from build123d import *

# Parameters (mm, degrees)
SKETCH_1_W          = 48
SKETCH_1_H          = 22
EXTRUDE_1_DEPTH     = 6
SKETCH_4_W          = 46
SKETCH_4_H          = 4
CUT_EXTRUDE_2_DEPTH = 22
SKETCH_5_W          = 42
SKETCH_5_H          = 1
CUT_EXTRUDE_3_DEPTH = 22
SKETCH_9_W          = 12
SKETCH_9_H          = 4.5
CUT_EXTRUDE_5_DEPTH = 6
SKETCH_10_W         = 6
SKETCH_10_H         = 3
EXTRUDE_2_DEPTH     = 6
SKETCH_11_W         = 6
SKETCH_11_H         = 3
EXTRUDE_3_DEPTH     = 6
SKETCH_12_R         = 1.5
CUT_EXTRUDE_6_DEPTH = 3
SKETCH_14_R         = 1.5
CUT_EXTRUDE_7_DEPTH = 3


with BuildPart() as part:
    # 草圖1 → 填料-伸長1 (new body)
    with BuildSketch(Plane.XY):
        with Locations((-24, -11)):
            Rectangle(SKETCH_1_W, SKETCH_1_H)
    extrude(amount=EXTRUDE_1_DEPTH)

    # 草圖4 → 除料-伸長2 (cut)
    with BuildSketch(Plane(origin=(0, 0, 0), x_dir=(1, 0, 0), z_dir=(0, 1, 0))):
        with Locations((-24, -3)):
            Rectangle(SKETCH_4_W, SKETCH_4_H)
    extrude(amount=-CUT_EXTRUDE_2_DEPTH, mode=Mode.SUBTRACT)

    # 草圖5 → 除料-伸長3 (cut)
    with BuildSketch(Plane(origin=(0, 0, 0), x_dir=(1, 0, 0), z_dir=(0, 1, 0))):
        with Locations((-24, -0.5)):
            Rectangle(SKETCH_5_W, SKETCH_5_H)
    extrude(amount=-CUT_EXTRUDE_3_DEPTH, mode=Mode.SUBTRACT)

    # 草圖9 → 除料-伸長5 (cut)
    with BuildSketch(Plane.XY.offset(6)):
        with Locations((-24, -19.75)):
            Rectangle(SKETCH_9_W, SKETCH_9_H)
    extrude(amount=-CUT_EXTRUDE_5_DEPTH, mode=Mode.SUBTRACT)

    # 草圖10 → 填料-伸長2 (add)
    with BuildSketch(Plane(origin=(0, 0, 0), x_dir=(0, 0, -1), z_dir=(1, 0, 0))):
        with Locations((-3, -20.5)):
            Rectangle(SKETCH_10_W, SKETCH_10_H)
    extrude(amount=EXTRUDE_2_DEPTH)

    # 草圖11 → 填料-伸長3 (add)
    with BuildSketch(Plane.ZY.offset(48)):
        with Locations((3, -20.5)):
            Rectangle(SKETCH_11_W, SKETCH_11_H)
    extrude(amount=EXTRUDE_3_DEPTH)

    # 草圖12 → 除料-伸長6 (cut)
    with BuildSketch(Plane(origin=(0, -19, 0), x_dir=(1, 0, 0), z_dir=(0, 1, 0))):
        with Locations(Location((3, -3, 0), (0, 0, 180))):
            Circle(SKETCH_12_R)
    extrude(amount=-CUT_EXTRUDE_6_DEPTH, mode=Mode.SUBTRACT)

    # 草圖14 → 除料-伸長7 (cut)
    with BuildSketch(Plane(origin=(0, -19, 0), x_dir=(1, 0, 0), z_dir=(0, 1, 0))):
        with Locations(Location((-51, -3, 0), (0, 0, 270))):
            Circle(SKETCH_14_R)
    extrude(amount=-CUT_EXTRUDE_7_DEPTH, mode=Mode.SUBTRACT)


solid = part.part
Work out the finished part from the listing and answer in its coordinate system (mm). A direction names the side the tool comes from. Give positions to 0.01 mm unless a question says otherwise; leave off trailing zeros. Order: outer loops, then holes, each group sorted by start corner. A loop starts at its lowest first (then second) coordinate and runs counter-clockwise, first axis right, second up. Notation, with made-up numbers: M -34,-11 L -21,-11 A34 cw -21,22 Z; hole C -1,2.5 d1. An arc over 180 degrees is marked long. Return JSON: item names as keys, results as strings.
Q1. The mould has two halves that part along Z. Classify faces 4 (the face through (-47, -14, 0)), 5 (the face through (-2, -11, 1)), 6 (the face through (-47, -11, 3)), 7 (the face through (-27.7, 0, 5.4)): pulls with the +Z half, pulls with the -Z half, needs draft (parallel to the pull), parting line crosses it, or undercut.
Answer below:
{"face 4": "pulls with the -Z half", "face 5": "undercut", "face 6": "undercut", "face 7": "needs draft"}
Q2. Find the intervals of material crossed by line 1 along X through (y, z) = (-19.75, 3.1); line 2 along X through (y, z) = (-15.25, 1.4); line 3 along Z through (x, y) = (-1.5, -3.25), in increasing order. Write a range as [from, to].
Answer below:
{"line 1": "x = [-54, -52.5], [-49.5, -47], [-1, 1.5], [4.5, 6]", "line 2": "x = [-48, -47], [-1, 0]", "line 3": "z = [0, 1], [5, 6]"}
Q3. Find section C-C, the plane y = -5. Write down the section's boundary in (x, z), and give its area (3 significant figures).
Answer below:
{"outline": "M -48,0 L -45,0 L -45,1 L -47,1 L -47,5 L -1,5 L -1,1 L -3,1 L -3,0 L 0,0 L 0,6 L -48,6 Z", "area": "62.0 mm^2"}
Q4. Find section B-B, the plane x = 3. Write down the section's boundary in (y, z).
Answer below:
{"outline": "M -22,0 L -19,0 L -19,1.5 L -22,1.5 Z; M -22,4.5 L -19,4.5 L -19,6 L -22,6 Z"}
Q5. Which of the six approach directions +Z, -Z, +X, -X, +Y, -Y give full straight-line access (tool end or side, diameter ignored) to faces 1 (the face through (-49.6, -19, 1.6)), 2 (the face through (-3, -10.8, 0.5)), 3 (the face through (-18, -19.8, 5.5))?
Answer below:
{"face 1": "+Z, -Z, -X, +Y", "face 2": "-Z, +Y, -Y", "face 3": "+Z, -Z, -Y"}
Q6. Each of these flat-tipped pins is pushed along its axis until it touches: pin 1 (2 mm diameter, centred on y = -13.5, z = 2, fed in from -X); pin 2 (6.5 mm diameter, centred on x = -23, y = -13.5, fed in from -Z); pin 3 (0.5 mm diameter, centred on y = -9, z = 0.5, fed in from +X); pin 4 (2.5 mm diameter, centred on x = -51, z = 3, fed in from -Y). Where does it stop, or does it pass through?
Answer below:
{"pin 1": "stops at x = -48", "pin 2": "stops at z = 5", "pin 3": "stops at x = 0", "pin 4": "passes through"}
Q7. Find section D-D, the plane x = -21.5. Write down the section's boundary in (y, z), and give its area (3 significant figures).
Answer below:
{"outline": "M -17.5,5 L 0,5 L 0,6 L -17.5,6 Z", "area": "17.5 mm^2"}
Q8. Find section A-A, the plane z = 3. Write down the section's boundary in (x, y).
Answer below:
{"outline": "M -54,-22 L -52.5,-22 L -52.5,-19 L -54,-19 Z; M -49.5,-22 L -47,-22 L -47,0 L -48,0 L -48,-19 L -49.5,-19 Z; M -1,-22 L 1.5,-22 L 1.5,-19 L 0,-19 L 0,0 L -1,0 Z; M 4.5,-22 L 6,-22 L 6,-19 L 4.5,-19 Z"}
